Build history of the part. All positions in model axes, mm. Face numbers are marked on the shaded views. A direction names the side the tool comes from. Round coordinates to 2 decimals unless told otherwise and drop trailing zeros. Write each loop counter-clockwise with the first axis right and the second up, starting at its lowest first coordinate (ties: lowest second). Pieces come first, ordered by that corner, then holes.
Item 1: 3-axis set-ups, long thin cutter, end or side, ignore diameter. For the marked faces 5, 6 and 7: which of +Z, -Z, +X, -X, +Y, -Y reach the whole face in a straight line?
Item 2: Mould opens along X. For the marked faces 1, 2, 3 and 4 say: +X half, -X half, draft (parallel to the pull), parting line (faces both ways), or undercut.
Item 3: Band-saw the part on A-A, the plane x = 40. Write the cut outline in (y, z).
Item 4: Drop flat-ended pins along their axis: pin 1 Ø4 at (x, y) = (5.5, -5.5) entering from -Z; pin 2 Ø9.5 at (y, z) = (4, 2.5) entering from +X; pin 3 Ø5 at (x, y) = (7, -3) entering from -Z; pin 4 Ø1 at (y, z) = (4, 6.5) entering from +X. Give the stop position or say it passes through.
Item 5: Wall check: probe 1 along Y at (x, z) = (2.65, 0); probe 2 along X at (y, z) = (0, 8). Give the ranges that are in metal, low to high.
```python
from build123d import *

# Parameters (mm, degrees)
FILETE1_R = 0.5
FILETE2_R = 0.5
FILETE3_R = 0.5
FILETE4_R = 0.5


with BuildPart() as part:
    # Esboço1 → Revolução1 (revolve)
    with BuildSketch(Plane.XY):
        Polygon((0, 5), (0, 9.54375), (8, 9.54375), (8, 7.14375), (10.62, 7.14375), (10.62, 9.54375), (12.62, 9.54375), (12.62, 3.96875), (42.62, 3.96875), (42.62, 0), (9.386751346, 0), (6.5, 5), align=None)
    revolve(axis=Axis((42.62, 0, 0), (-1, 0, 0)))

    # Filete1
    filete1_edges = [part.edges().sort_by_distance(p)[0] for p in [
        (42.62, -3.96875, 0),
    ]]
    fillet(filete1_edges, radius=FILETE1_R)

    # Filete2
    filete2_edges = [part.edges().sort_by_distance(p)[0] for p in [
        (0, -5, 0),
    ]]
    fillet(filete2_edges, radius=FILETE2_R)

    # Filete3
    filete3_edges = [part.edges().sort_by_distance(p)[0] for p in [
        (0, -9.54375, 0),
    ]]
    fillet(filete3_edges, radius=FILETE3_R)

    # Filete4
    filete4_edges = [part.edges().sort_by_distance(p)[0] for p in [
        (12.62, -9.54375, 0),
    ]]
    fillet(filete4_edges, radius=FILETE4_R)


solid = part.part
```
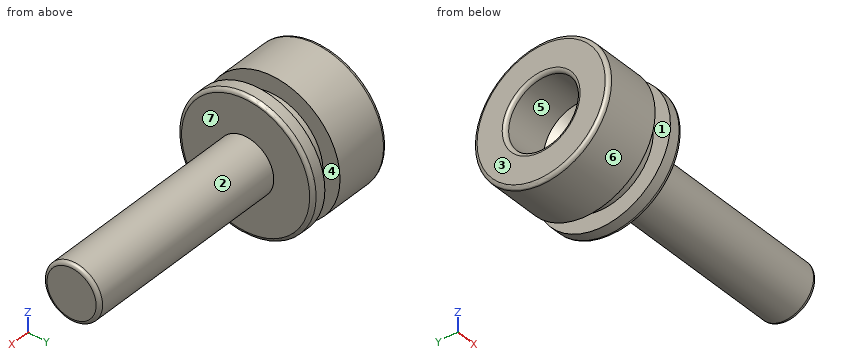
Results:
1. face 5: -X
1. face 6: +X, -X
1. face 7: +X
2. face 1: undercut
2. face 2: draft
2. face 3: -X half
2. face 4: undercut
3. outline: circle Ø7.94 at (0, 0)
4. pin 1: stops at z = -8.88
4. pin 2: stops at x = 42.62
4. pin 3: stops at z = -9.53
4. pin 4: stops at x = 12.62
5. probe 1: y = -9.54 to -5, 5 to 9.54
5. probe 2: x = 0 to 8, 10.62 to 12.62
